Autodesk Inventor part; units mm, degrees
ref_plane "YZ Plane" through (0, 0, 0) normal (1, 0, 0) x (0, 1, 0)
ref_plane "XZ Plane" through (0, 0, 0) normal (0, 1, 0) x (-1, 0, 0)
ref_plane "XY Plane" through (0, 0, 0) normal (0, 0, 1) x (1, 0, 0)
sketch "Sketch1" plane through (0, 0, 0) normal (0, 0, 1) x (1, 0, 0)
  line L0 (-76.2, -25.4) -> (76.2, -25.4)
  line L1 (76.2, -25.4) -> (76.2, 25.4)
  line L2 (76.2, 25.4) -> (-76.2, 25.4)
  line L3 (-76.2, 25.4) -> (-76.2, -25.4)
  line L4 (-76.2, -25.4) -> (76.2, 25.4) construction
  line L5 (76.2, -25.4) -> (-76.2, 25.4) construction
  point P0 (0, 0)
  dimension "d0" = 152.4
  dimension "d1" = 50.8
extrude "Extrusion1" add sketch "Sketch1" along normal blind 6.35
sketch "Sketch2" plane through (0, 0, 6.35) normal (0, 0, 1) x (1, 0, 0)
  line L0 (-76.2, 25.4) -> (-76.2, -25.4)
  line L1 (-63.5, 6.35) -> (-50.8, 6.35)
  line L2 (-50.8, 6.35) -> (-50.8, -6.35)
  line L3 (-50.8, -6.35) -> (-63.5, -6.35)
  line L4 (-63.5, -6.35) -> (-63.5, 6.35)
  point P0 (0, 0)
  dimension "d4" = 12.7
  dimension "d5" = 12.7
  dimension "d6" = 6.35
  dimension "d7" = 12.7
extrude "Extrusion2" add sketch "Sketch2" along normal blind 38.1
sketch "Sketch3" plane through (0, 0, 6.35) normal (0, 0, 1) x (1, 0, 0)
  line L0 (76.2, -25.4) -> (76.2, 25.4)
  line L1 (50.8, -6.35) -> (63.5, -6.35)
  line L2 (63.5, -6.35) -> (63.5, 6.35)
  line L3 (63.5, 6.35) -> (50.8, 6.35)
  line L4 (50.8, 6.35) -> (50.8, -6.35)
  point P0 (0, 0)
  dimension "d10" = 12.7
  dimension "d11" = 12.7
  dimension "d12" = 6.35
  dimension "d13" = 12.7
extrude "Extrusion3" add sketch "Sketch3" along normal blind 63.5
sketch "Sketch4" plane through (63.5, -6.35, 6.35) normal (1, 0, 0) x (0, 0, -1)
  circle A0 centre (-57.15, 6.35) radius 3.175
  line L0 (0, 12.7) -> (-63.5, 12.7)
  line L1 (-63.5, 0) -> (-63.5, 12.7)
  point P0 (6.35, 6.35)
  dimension "d16" = 6.35
  dimension "d19" = 6.35
  dimension "d20" = 6.35
extrude "Extrusion4" cut sketch "Sketch4" against normal through all
sketch "Sketch5" plane through (-50.8, -6.35, 6.35) normal (1, 0, 0) x (0, 0, -1)
  line L0 (0, 12.7) -> (-38.1, 12.7)
  line L1 (-38.1, 0) -> (-38.1, 12.7)
  circle A0 centre (-31.75, 6.35) radius 3.175
  point P0 (6.35, 6.35)
  dimension "d21" = 6.35
  dimension "d22" = 6.35
  dimension "d23" = 6.35
extrude "Extrusion5" cut sketch "Sketch5" against normal through all
equation "\"d5\" = d4"
properties part number "base" material "Silicon Nitride"
Check sheet for the modelled part. Datum: model origin and axes. Units: mm. A direction names the side the tool comes from. Give positions to 0.01 mm unless a question says otherwise; leave off trailing zeros. Write each loop counter-clockwise with the first axis right and the second up, starting at its lowest first coordinate (ties: lowest second). Pieces come first, ordered by that corner, then holes.
Item 1: Access from +Z, -Z, +X, -X, +Y, -Y to the whole of each face (thin tool, end or side, straight path). Record for faces 1 (the face through (-57, -6.35, 25)), 2 (the face through (-57.06, 0.14, 41.27)), 3 (the face through (-57, 0, 44.45)).
Item 2: Draft check along X on faces 4 (the face through (1, 25.4, 3)), 5 (the face through (76.2, 0, 3)), 6 (the face through (50.8, 0, 38)), 7 (the face through (-1, 0, 6.35)). Enter one of: released by +X, released by -X, zero draft, split by the parting line, or undercut.
Item 3: Gauge pin test, flat ends, axial feed: pin 1 (14 mm diameter, centred on x = 54.5, z = 45.5, fed in from +Y); pin 2 (8 mm diameter, centred on x = -53, z = 15, fed in from -Y); pin 3 (5 mm diameter, centred on y = 0, z = 38.1, fed in from -X). Record the tip position at first contact, or that the pin passes through.
Item 4: Cross-section at A-A (z = 15). Enter the section's corners in (x, y), and give its area (3 significant figures).
Item 5: Cross-section at D-D (z = 38.1). Enter the section's corners in (x, y) (3 decimals), and give its area (3 significant figures).
Item 6: Cross-section at B-B (y = 0). Enter the section's corners in (x, z) (3 decimals), and give its area (3 significant figures).
Item 7: Scan lines: L1, parallel to X at y = 3, z = 25; L2, parallel to Y at x = 60, z = 63.5 (3 decimals); L3, parallel to Z at x = 0, y = 12. Record each from-to range of solid material in increasing order.
Item 8: Cross-section at C-C (x = 60.5). Enter the section's corners in (y, z) (3 decimals).
Report:
1. face 1: +Z, +X, -X, -Y
1. face 2: -X
1. face 3: +Z, -X, +Y, -Y
2. face 4: zero draft
2. face 5: released by +X
2. face 6: undercut
2. face 7: undercut
3. pin 1: stops at y = 6.35
3. pin 2: stops at y = -6.35
3. pin 3: stops at x = 50.8
4. outline: (-63.5, -6.35) - (-50.8, -6.35) - (-50.8, 6.35) - (-63.5, 6.35) - close; (50.8, -6.35) - (63.5, -6.35) - (63.5, 6.35) - (50.8, 6.35) - close
4. area: 323 mm2
5. outline: (-63.5, -6.35) - (-50.8, -6.35) - (-50.8, -3.175) - (-63.5, -3.175) - close; (-63.5, 3.175) - (-50.8, 3.175) - (-50.8, 6.35) - (-63.5, 6.35) - close; (50.8, -6.35) - (63.5, -6.35) - (63.5, 6.35) - (50.8, 6.35) - close
5. area: 242 mm2
6. outline: (-76.2, 0) - (76.2, 0) - (76.2, 6.35) - (63.5, 6.35) - (63.5, 60.325) - (50.8, 60.325) - (50.8, 6.35) - (-50.8, 6.35) - (-50.8, 34.925) - (-63.5, 34.925) - (-63.5, 6.35) - (-76.2, 6.35) - close; (-63.5, 41.275) - (-50.8, 41.275) - (-50.8, 44.45) - (-63.5, 44.45) - close; (50.8, 66.675) - (63.5, 66.675) - (63.5, 69.85) - (50.8, 69.85) - close
6. area: 2,100 mm2
7. L1: x = -63.5 to -50.8, 50.8 to 63.5
7. L2: y = -6.35 to -3.175, 3.175 to 6.35
7. L3: z = 0 to 6.35
8. outline: (-25.4, 0) - (25.4, 0) - (25.4, 6.35) - (6.35, 6.35) - (6.35, 69.85) - (-6.35, 69.85) - (-6.35, 6.35) - (-25.4, 6.35) - close; hole circle Ø6.35 at (0, 63.5)
